Read the model definition and answer for the solid it produces. Units are mm, in the model's axes. Face numbers are marked on the shaded views. Give positions to 0.01 mm unless a question says otherwise; leave off trailing zeros. Order: outer loops, then holes, each group sorted by start corner. A loop starts at its lowest first (then second) coordinate and runs counter-clockwise, first axis right, second up. Notation, with made-up numbers: (18.5, 78.25) - (73.5, 78.25) arc R36 cw to (73.5, 115.25) - close; hole circle Ø1 at (87.25, 26). An arc over 180 degrees is marked (long way). Return JSON: item names as keys, results as strings.
Autodesk Inventor part; units mm, degrees
ref_plane "YZ Plane" through (0, 0, 0) normal (1, 0, 0) x (0, 1, 0)
ref_plane "XZ Plane" through (0, 0, 0) normal (0, 1, 0) x (-1, 0, 0)
ref_plane "XY Plane" through (0, 0, 0) normal (0, 0, 1) x (1, 0, 0)
ref_plane "Work Plane1" through (186.7197, -101.2807, 0) normal (0, 0, 1) x (1, 0, 0)
sketch "Sketch1" plane through (186.7197, -101.2807, 0) normal (0, 0, 1) x (1, 0, 0)
  line L0 (-168.7197, 119.2807) -> (-204.7197, 119.2807)
  line L1 (-204.7197, 119.2807) -> (-204.7197, 83.2807)
  line L2 (-204.7197, 83.2807) -> (-168.7197, 83.2807)
  line L3 (-168.7197, 83.2807) -> (-168.7197, 119.2807)
  point P0 (-186.7197, 101.2807)
  point P1 (-168.7197, 101.2807)
  point P2 (-186.7197, 83.2807)
  point P3 (-204.7197, 101.2807)
  dimension "d0" = 36
  dimension "d1" = 36
  dimension "d8" = 0
  dimension "d9" = 0
extrude "Extrusion1" add sketch "Sketch1" along normal blind 22
sketch "Sketch3" plane through (186.7197, -101.2807, 22) normal (0, 0, 1) x (1, 0, 0)
  circle A0 centre (-174.8697, 120.9651) radius 3.25
  circle A1 centre (-198.5697, 101.2807) radius 3.25
  line L0 (-211.9197, 101.2807) -> (-161.5197, 101.2807)
  circle A2 centre (-174.8697, 81.5964) radius 3.25
  line L1 (-174.8697, 120.9651) -> (-168.7197, 120.9651)
  line L2 (-168.7197, 83.2807) -> (-168.7197, 119.2807)
  line L3 (-198.5697, 101.2807) -> (-204.7197, 101.2807)
  line L4 (-204.7197, 119.2807) -> (-204.7197, 83.2807)
  point P0 (-186.7197, 101.2807)
  dimension "d10" = 6.5
  dimension "d11" = 6.5
  dimension "d12" = 23.7
hole "Hole1" at (11.85, -19.6844, 22) at (11.85, 19.6844, 22) at (-11.85, 0, 22) direction (0, 0, -1) diameter 6.5 depth 6
hole "Hole2" at (-11.85, 0, 22) at (11.85, -19.6844, 22) at (11.85, 19.6844, 22) direction (0, 0, -1) diameter 4 end through all
equation "\"d1\" = d0"
equation "\"d11\" = d10"
properties part number "Camera_mount"
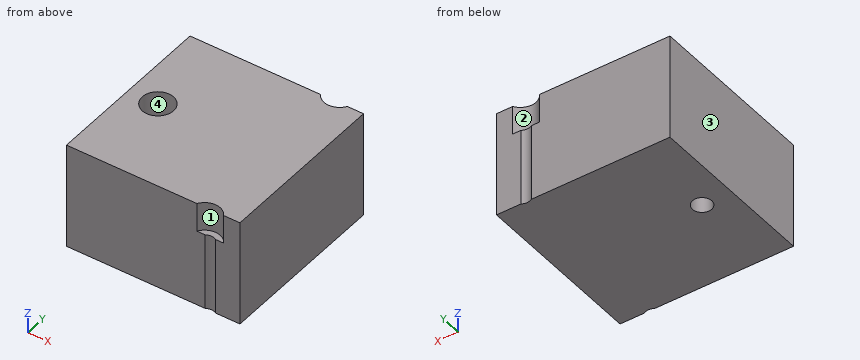
Q1. Given pin 1 (0.8 mm diameter, centred on x = 11.5, y = -17, fed in from +Z), flat-ended and moving along its own axis, determine where the tip first touches the part or whether it passes through.
Values:
{"pin 1": "stops at z = 16"}
Q2. Determine the mould class of the marked faces 1, 2, 3 and 4 for opening direction Y: released by +Y, released by -Y, zero draft, split by the parting line, or undercut.
Values:
{"face 1": "released by -Y", "face 2": "released by +Y", "face 3": "zero draft", "face 4": "undercut"}
Q3. Consider L1, parallel to X at y = 0, z = 12.25; L2, parallel to Y at x = -11.85, z = 20.7; L3, parallel to Y at x = -11.85, z = 4. Determine where each line is inside the solid, lowest interval first.
Values:
{"L1": "x = -18 to -13.85, -9.85 to 18", "L2": "y = -18 to -3.25, 3.25 to 18", "L3": "y = -18 to -2, 2 to 18"}
Q4. A cutting plane is placed at C-C (z = 20.75). Write down the section's boundary in (x, y), and give its area (3 significant figures).
Values:
{"outline": "(-18, -18) - (9.07, -18) arc R3.25 cw to (14.63, -18) - (18, -18) - (18, 18) - (14.63, 18) arc R3.25 cw to (9.07, 18) - (-18, 18) - close; hole circle Ø6.5 at (-11.85, 0)", "area": "1,250 mm²"}
Q5. A cutting plane is placed at B-B (y = 0). Write down the section's boundary in (x, z).
Values:
{"outline": "(-18, 0) - (-13.85, 0) - (-13.85, 16) - (-15.1, 16) - (-15.1, 22) - (-18, 22) - close; (-9.85, 0) - (18, 0) - (18, 22) - (-8.6, 22) - (-8.6, 16) - (-9.85, 16) - close"}
Q6. A cutting plane is placed at A-A (x = -11.85). Write down the section's boundary in (y, z).
Values:
{"outline": "(-18, 0) - (-2, 0) - (-2, 16) - (-3.25, 16) - (-3.25, 22) - (-18, 22) - close; (2, 0) - (18, 0) - (18, 22) - (3.25, 22) - (3.25, 16) - (2, 16) - close"}
